Design review of the part built by this model. Coordinates are the model's own, in mm. Face numbers are marked on the shaded views. Give positions to 0.01 mm unless a question says otherwise; leave off trailing zeros. Loops run counter-clockwise (first coordinate to the right, second up) from the corner with the lowest first, then second, coordinate; pieces in that order, holes last. Notation, with made-up numbers: M 0,84.25 L 54,84.25 A10 cw 54,100.25 Z; hole C 10.25,-33.75 d6. An arc over 180 degrees is marked long. Answer as CSV lines item,"result".
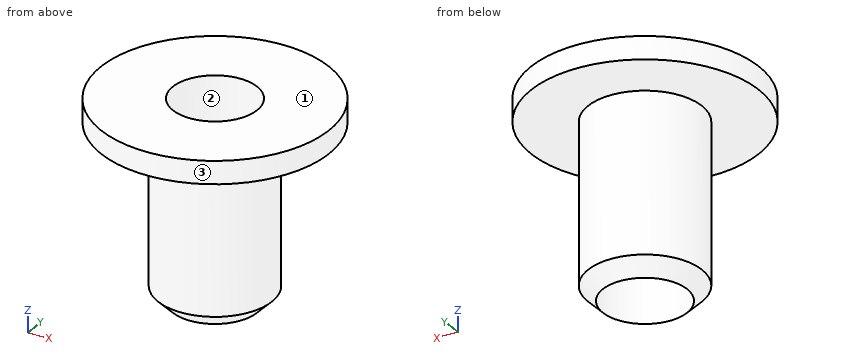
```python
from build123d import *

# Parameters (mm, degrees)
ESQUISSE1_R             = 15
BOSS_EXTRU_1_DEPTH      = 3
ESQUISSE2_R             = 7.5
BOSS_EXTRU_2_DEPTH      = 23
CHANFREIN1_SIZE         = 2
ESQUISSE3_R             = 5.55
ENL_V_MAT_EXTRU_1_DEPTH = 23
ESQUISSE4_R             = 5.55
ENL_V_MAT_EXTRU_2_DEPTH = 26


with BuildPart() as part:
    # Esquisse1 → Boss.-Extru.1 (new body)
    with BuildSketch(Plane.XY):
        Circle(ESQUISSE1_R)
    extrude(amount=BOSS_EXTRU_1_DEPTH)

    # Esquisse2 → Boss.-Extru.2 (add)
    with BuildSketch(Plane(origin=(0, 0, 0), x_dir=(-1, 0, 0), z_dir=(0, 0, -1))):
        Circle(ESQUISSE2_R)
    extrude(amount=BOSS_EXTRU_2_DEPTH)

    # Chanfrein1
    chanfrein1_edges = [part.edges().sort_by_distance(p)[0] for p in [
        (7.5, 0, -23),
    ]]
    chamfer(chanfrein1_edges, length=CHANFREIN1_SIZE)

    # Esquisse3 → Enlèv. mat.-Extru.1 (cut)
    with BuildSketch(Plane(origin=(0, 0, -23), x_dir=(-1, 0, 0), z_dir=(0, 0, -1))):
        Circle(ESQUISSE3_R)
    extrude(amount=-ENL_V_MAT_EXTRU_1_DEPTH, mode=Mode.SUBTRACT)

    # Esquisse4 → Enlèv. mat.-Extru.2 (cut)
    with BuildSketch(Plane.XY.offset(3)):
        Circle(ESQUISSE4_R)
    extrude(amount=-ENL_V_MAT_EXTRU_2_DEPTH, mode=Mode.SUBTRACT)


solid = part.part
```
1. The part is to be moulded in two halves that separate along Y. For the marked faces 1, 2 and 3, say which applies: pulls with the +Y half, pulls with the -Y half, needs draft (parallel to the pull), parting line crosses it, or undercut.
Answer block:
face 1,"needs draft"
face 2,"undercut"
face 3,"parting line crosses it"
2. We need section A-A, the plane y = 0. Write out the cut boundary in (x, z), plus the area to 3 significant figures.
Answer block:
outline,"M -15,0 L -7.5,0 L -7.5,-21 L -5.55,-22.95 L -5.55,3 L -15,3 Z; M 5.55,-22.95 L 7.5,-21 L 7.5,0 L 15,0 L 15,3 L 5.55,3 Z"
area,"142 mm²"
3. We need section D-D, the plane y = 12. Write out the cut boundary in (x, z), plus the area to 3 significant figures.
Answer block:
outline,"M -9,0 L 9,0 L 9,3 L -9,3 Z"
area,"54.0 mm²"
4. For P1, Ø6, axis at x = 8.5, z = -6.5, coming from the -Y side; P2, Ø3, axis at x = -0.5, z = -9.5, coming from the +Y side; P3, Ø8, axis at y = 3.5, z = -18, coming from the +X side, all flat-tipped, find the tip position at first contact; note any pin that passes through.
Answer block:
P1,"y = -5.1"
P2,"y = 7.5"
P3,"x = 7.5"
5. We need section C-C, the plane z = -14.5. Write out the cut boundary in (x, y).
Answer block:
outline,"C 0,0 d15; hole C 0,0 d11.1"
6. To check wall thickness, follow L1, parallel to Y at x = 0, z = -5.5; L2, parallel to Z at x = 5, y = 8; L3, parallel to Y at x = -3.25, z = -1. State the ranges of each line that lie inside material, in increasing order. Write a range as [from, to].
Answer block:
L1,"[-7.5, -5.55], [5.55, 7.5]"
L2,"[0, 3]"
L3,"[-6.76, -4.5], [4.5, 6.76]"
